For this review, take the finished solid that the model builds, in its own axes (mm). A direction names the side the tool comes from. Coordinates: 2 decimals unless noted, no trailing zeros. Loops run counter-clockwise (first coordinate to the right, second up) from the corner with the lowest first, then second, coordinate; pieces in that order, holes last. Notation, with made-up numbers: (6, 27) -> (33, 27) arc R16 cw to (33, 39) -> close; hole circle Ø10 at (57.5, 3.5). An arc over 180 degrees is marked (long way). Answer in a Markdown table with one row per item.
Autodesk Fusion 360 part; units mm, degrees
sketch "Sketch1" plane through (0, 0, 0) normal (0, 1, 0) x (1, 0, 0)
  line L0 (0, 0) -> (38, 0)
  line L1 (38, 0) -> (38, 14)
  line L2 (38, 14) -> (0, 14)
  line L3 (0, 14) -> (0, 0)
  line L4 (3.9603, 3.1256) -> (35.9564, 3.1256) construction
  line L5 (35.9564, 3.1256) -> (35.9564, 11.1256) construction
  line L6 (35.9564, 11.1256) -> (3.9603, 11.1256) construction
  line L7 (3.9603, 11.1256) -> (3.9603, 3.1256) construction
  dimension "d1" = 14
  dimension "d2" = 38
extrude "Extrude1" add sketch "Sketch1" against normal blind 6
cylinder "CylinderPrimitive1" add diameter 2 height 3 placed x (0, 0, -1) y (0, 1, 0) z (1, 0, 0) at (38, -3, -2.4977)
sketch "Sketch3" plane through (38, 0, 0) normal (1, 0, 0) x (0, 0, -1)
  circle A0 centre (2.4977, -3) radius 1
  line L0 (14, 0) -> (0, 0)
  line L1 (0, 0) -> (0, -6)
  line L2 (0, -6) -> (14, -6)
  line L3 (14, -6) -> (14, 0)
cylinder "CylinderPrimitive2" add diameter 2 height 3 placed x (0, 0, -1) y (0, 1, 0) z (1, 0, 0) at (38, -3, -7)
cylinder "CylinderPrimitive3" add diameter 2 height 3 placed x (0, 0, -1) y (0, 1, 0) z (1, 0, 0) at (38, -3.0833, -11.2079)
sketch "Sketch5" plane through (0, 0, 0) normal (-1, 0, 0) x (0, 0, 1)
  line L0 (0, 0) -> (-14, 0)
  line L1 (-14, 0) -> (-14, -6)
  line L2 (-14, -6) -> (0, -6)
  line L3 (0, -6) -> (0, 0)
cylinder "CylinderPrimitive4" add diameter 2 height 3 placed x (0, 0, 1) y (0, 1, 0) z (-1, 0, 0) at (0, -3, -12.5)
cylinder "CylinderPrimitive5" add diameter 2 height 3 placed x (0, 0, 1) y (0, 1, 0) z (-1, 0, 0) at (0, -3, -1.6)
cylinder "CylinderPrimitive6" add diameter 1 height 3 placed x (0, 0, 1) y (0, 1, 0) z (-1, 0, 0) at (0, -3, -10)
cylinder "CylinderPrimitive7" add diameter 1 height 3 placed x (0, 0, 1) y (0, 1, 0) z (-1, 0, 0) at (0, -3, -8.5)
cylinder "CylinderPrimitive8" add diameter 1 height 3 placed x (0, 0, 1) y (0, 1, 0) z (-1, 0, 0) at (0, -3, -7)
Item 1: Take a section at A-A, the plane z = -7. State the section outline as (x, y) points, and give its area (3 significant figures).
Worked answers:
| item | result |
|---|---|
| outline | (-3, -3.5) -> (0, -3.5) -> (0, -6) -> (38, -6) -> (38, -4) -> (41, -4) -> (41, -2) -> (38, -2) -> (38, 0) -> (0, 0) -> (0, -2.5) -> (-3, -2.5) -> close |
| area | 237 mm² |
Item 2: Take a section at C-C, the plane z = -11. State the section outline as (x, y) points, and give its area (3 significant figures).
Worked answers:
| item | result |
|---|---|
| outline | (0, -6) -> (38, -6) -> (38, -4.06) -> (41, -4.06) -> (41, -2.11) -> (38, -2.11) -> (38, 0) -> (0, 0) -> close |
| area | 234 mm² |
Item 3: For L1, parallel to X at y = -0.5, z = -12.75; L2, parallel to X at y = -3.6, z = -6.25, list the stretches that pass through material, from the lowest coordinate up.
Worked answers:
| item | result |
|---|---|
| L1 | 0 to 38 |
| L2 | 0 to 41 |
Item 4: Insertion check: pin 1 (3 mm diameter, centred on x = 4.5, z = -11.5, fed in from +Y); pin 2 (2 mm diameter, centred on y = -2, z = -5, fed in from +X). Each pin has a flat end and moves straight along its axis. Give the tip position at first contact, or say it passes through.
Worked answers:
| item | result |
|---|---|
| pin 1 | y = 0 |
| pin 2 | x = 38 |
Item 5: For faces 1 (the cylindrical face through (39.52, -2.41, -10.47)), 2 (the flat face through (-3, -3, -8.5)), 3 (the cylindrical face through (-1.5, -2.7, -10.4)), list the 3-axis set-ups (+Z, -Z, +X, -X, +Y, -Y) from which the entire face can be reached by the end or side of a thin tool; tool diameter is ignored.
Worked answers:
| item | result |
|---|---|
| face 1 | +X |
| face 2 | +Z, -Z, -X, +Y, -Y |
| face 3 | -X |
Item 6: Take a section at B-B, the plane y = -1.5. State the section outline as (x, z) points, and give its area (3 significant figures).
Worked answers:
| item | result |
|---|---|
| outline | (0, -14) -> (38, -14) -> (38, 0) -> (0, 0) -> close |
| area | 532 mm² |
